from build123d import *

# Parameters (mm, degrees)
ESBO_O1_W                = 175
ESBO_O1_H                = 95
RESSALTO_EXTRUS_O1_DEPTH = 10
ESBO_O2_W                = 6
ESBO_O2_H                = 30
RESSALTO_EXTRUS_O2_DEPTH = 10
ESBO_O3_W                = 6
ESBO_O3_H                = 30
RESSALTO_EXTRUS_O3_DEPTH = 10
ESBO_O4_W                = 30
ESBO_O4_H                = 6
RESSALTO_EXTRUS_O4_DEPTH = 10
ESBO_O5_W                = 30
ESBO_O5_H                = 6
RESSALTO_EXTRUS_O5_DEPTH = 10
CORTE_EXTRUS_O1_DEPTH    = 10


with BuildPart() as part:
    # Esboço1 → Ressalto-extrusão1 (new body)
    with BuildSketch(Plane.XY):
        Rectangle(ESBO_O1_W, ESBO_O1_H)
    extrude(amount=RESSALTO_EXTRUS_O1_DEPTH)

    # Esboço2 → Ressalto-extrusão2 (add)
    with BuildSketch(Plane.ZY.offset(87.5)):
        with Locations((5, 0)):
            Rectangle(ESBO_O2_W, ESBO_O2_H)
    extrude(amount=RESSALTO_EXTRUS_O2_DEPTH)

    # Esboço3 → Ressalto-extrusão3 (add)
    with BuildSketch(Plane(origin=(87.5, 0, 0), x_dir=(0, 0, -1), z_dir=(1, 0, 0))):
        with Locations((-5, 0)):
            Rectangle(ESBO_O3_W, ESBO_O3_H)
    extrude(amount=RESSALTO_EXTRUS_O3_DEPTH)

    # Esboço4 → Ressalto-extrusão4 (add)
    with BuildSketch(Plane.XZ.offset(47.5)):
        with Locations((37.5, 5)):
            Rectangle(ESBO_O4_W, ESBO_O4_H)
        with Locations((-37.5, 5)):
            Rectangle(ESBO_O4_W, ESBO_O4_H)
    extrude(amount=RESSALTO_EXTRUS_O4_DEPTH)

    # Esboço5 → Ressalto-extrusão5 (add)
    with BuildSketch(Plane(origin=(0, 47.5, 0), x_dir=(1, 0, 0), z_dir=(0, 1, 0))):
        with Locations((0, -5)):
            Rectangle(ESBO_O5_W, ESBO_O5_H)
    extrude(amount=RESSALTO_EXTRUS_O5_DEPTH)

    # Esboço6 → Corte-extrusão1 (cut)
    with BuildSketch(Plane.XY.offset(10)):
        with BuildLine():
            Line((-77.5, -35), (-72.5, 35))
            ThreePointArc((-72.5, 35), (-70, 35.877501001), (-67.5, 35))
            Line((-67.5, 35), (-72.5, -35))
            ThreePointArc((-72.5, -35), (-75, -35.877501001), (-77.5, -35))
        make_face()
        with BuildLine():
            Line((-62.5, -35), (-57.5, 35))
            ThreePointArc((-57.5, 35), (-60, 35.877501001), (-62.5, 35))
            Line((-62.5, 35), (-67.5, -35))
            ThreePointArc((-67.5, -35), (-65, -35.877501001), (-62.5, -35))
        make_face()
        with BuildLine():
            Line((-52.5, -35), (-47.5, 35))
            ThreePointArc((-47.5, 35), (-50, 35.877501001), (-52.5, 35))
            Line((-52.5, 35), (-57.5, -35))
            ThreePointArc((-57.5, -35), (-55, -35.877501001), (-52.5, -35))
        make_face()
        with BuildLine():
            Line((-42.5, -35), (-37.5, 35))
            ThreePointArc((-37.5, 35), (-40, 35.877501001), (-42.5, 35))
            Line((-42.5, 35), (-47.5, -35))
            ThreePointArc((-47.5, -35), (-45, -35.877501001), (-42.5, -35))
        make_face()
        with BuildLine():
            Line((-32.5, -35), (-27.5, 35))
            ThreePointArc((-27.5, 35), (-30, 35.877501001), (-32.5, 35))
            Line((-32.5, 35), (-37.5, -35))
            ThreePointArc((-37.5, -35), (-35, -35.877501001), (-32.5, -35))
        make_face()
        with BuildLine():
            Line((-22.5, -35), (-17.5, 35))
            ThreePointArc((-17.5, 35), (-20, 35.877501001), (-22.5, 35))
            Line((-22.5, 35), (-27.5, -35))
            ThreePointArc((-27.5, -35), (-25, -35.877501001), (-22.5, -35))
        make_face()
        with BuildLine():
            Line((-12.5, -35), (-7.5, 35))
            ThreePointArc((-7.5, 35), (-10, 35.877501001), (-12.5, 35))
            Line((-12.5, 35), (-17.5, -35))
            ThreePointArc((-17.5, -35), (-15, -35.877501001), (-12.5, -35))
        make_face()
        with BuildLine():
            Line((-2.5, -35), (2.5, 35))
            ThreePointArc((2.5, 35), (0, 35.877501001), (-2.5, 35))
            Line((-2.5, 35), (-7.5, -35))
            ThreePointArc((-7.5, -35), (-5, -35.877501001), (-2.5, -35))
        make_face()
        with BuildLine():
            Line((7.5, -35), (12.5, 35))
            ThreePointArc((12.5, 35), (10, 35.877501001), (7.5, 35))
            Line((7.5, 35), (2.5, -35))
            ThreePointArc((2.5, -35), (5, -35.877501001), (7.5, -35))
        make_face()
    extrude(amount=-CORTE_EXTRUS_O1_DEPTH, mode=Mode.SUBTRACT)


solid = part.part
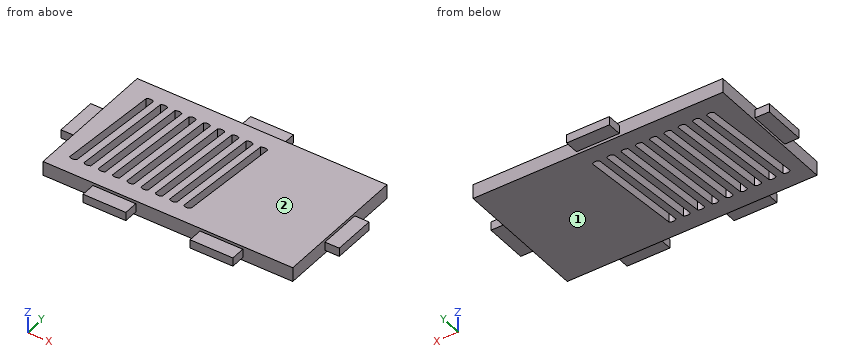
Design review of the part built by this model. Coordinates are the model's own, in mm. Face numbers are marked on the shaded views. Coordinates: 2 decimals unless noted, no trailing zeros. Order: outer loops, then holes, each group sorted by start corner. A loop starts at its lowest first (then second) coordinate and runs counter-clockwise, first axis right, second up.
Item 1: For line 1 (X direction, y = -49, z = 7.75); line 2 (X direction, y = -47, z = 2.5); line 3 (Y direction, x = 37.5, z = 9), list the stretches that pass through material, from the lowest coordinate up.
Item 2: For pin 1 Ø5 at (y, z) = (-53.5, 5.5) entering from -X; pin 2 Ø3 at (y, z) = (54.5, 6) entering from -X; pin 3 Ø5 at (x, y) = (-91.5, 1.5) entering from -Z, all flat-tipped, find the tip position at first contact; note any pin that passes through.
Item 3: Take a section at B-B, the plane z = 5.25. Count the separate pieces of the cut face and the enclosed holes in it, then the cut area to 3 significant figures.
Item 4: Take a section at A-A, the plane x = -29.5. Write out the cut boundary in (y, z), then the cut area to 3 significant figures.
Item 5: Take a section at D-D, the plane y = 39.5. Write out the cut boundary in (x, z), then the cut area to 3 significant figures.
Item 6: The part is to be moulded in two halves that separate along Z. For the marked faces 1 and 2, say which applies: pulls with the +Z half, pulls with the -Z half, needs draft (parallel to the pull), parting line crosses it, or undercut.
The answers:
1. line 1: x = -52.5 to -22.5, 22.5 to 52.5
1. line 2: x = -87.5 to 87.5
1. line 3: y = -47.5 to 47.5
2. pin 1: stops at x = -52.5
2. pin 2: stops at x = -15
2. pin 3: stops at z = 2
3. separate pieces: 1
3. enclosed holes: 9
3. area: 14,900 mm2
4. outline: (-57.5, 2) - (-47.5, 2) - (-47.5, 0) - (7, 0) - (7, 10) - (-47.5, 10) - (-47.5, 8) - (-57.5, 8) - close; (35.85, 0) - (47.5, 0) - (47.5, 10) - (35.85, 10) - close
4. area: 722 mm2
5. outline: (-87.5, 0) - (87.5, 0) - (87.5, 10) - (-87.5, 10) - close
5. area: 1,750 mm2
6. face 1: pulls with the -Z half
6. face 2: pulls with the +Z half
